Design review of the part shown in the three views and the two pictorial views. Dimensions are in mm from the part's minimum x, y and z. Coordinates: 2 decimals unless noted, no trailing zeros. Loops run counter-clockwise (first coordinate to the right, second up) from the corner with the lowest first, then second, coordinate; pieces in that order, holes last. Notation, with made-up numbers: M 55,-17.5 L 66,-17.5 A16 ccw 66,8.5 Z; hole C -20.5,-0.75 d4. An arc over 180 degrees is marked long. Use one line per item in the form item = value.
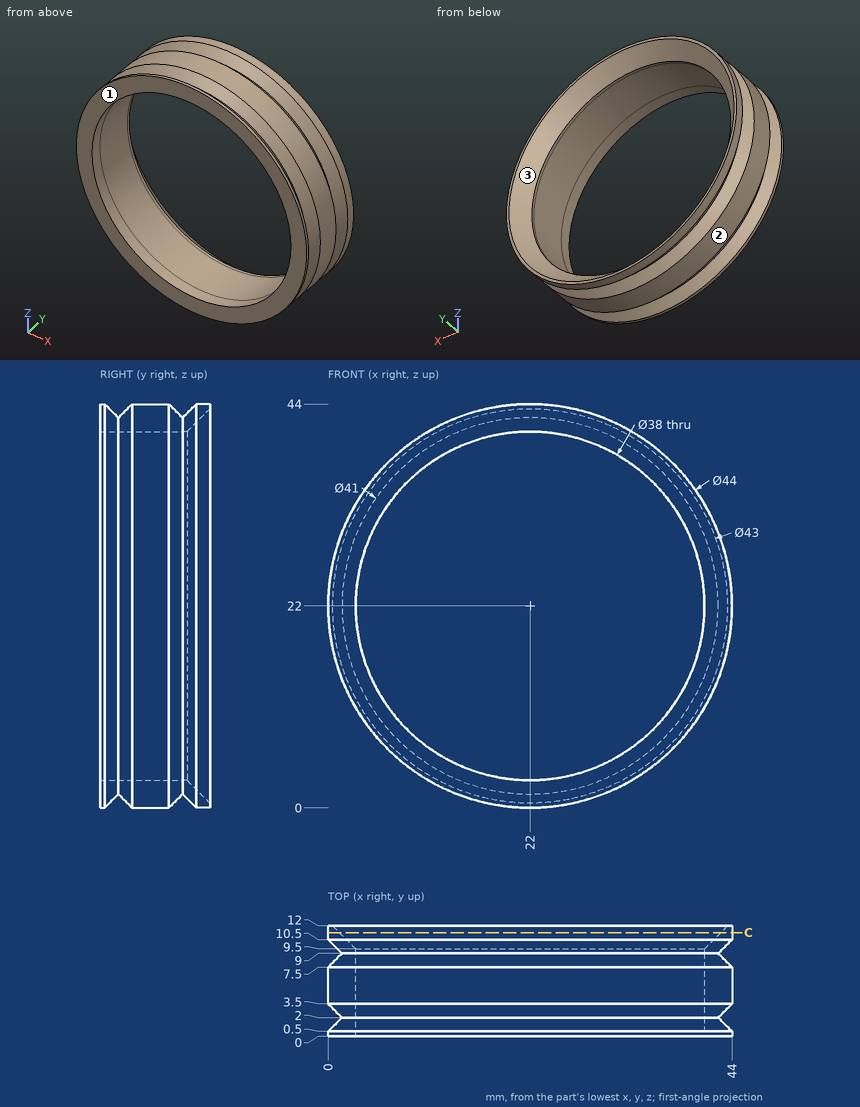
1. Add section C-C (y = 11.25). State the section outline as (x, z) points, then the cut area to 3 significant figures.
Response values:
outline = C 22,22 d44; hole C 22,22 d41.5
area = 168 mm^2
2. Wall thickness on line 1 along Z through (x, y) = (22, 6.5); line 2 along X through (y, z) = (2.25, 16); line 3 along X through (y, z) = (7.25, 21): over which ranges is each line inside the solid? List them lowest first. Write a range as from..to.
Response values:
line_1 = 0..3, 41..44
line_2 = 2.14..3.97, 40.03..41.86
line_3 = 0.02..3.03, 40.97..43.98
3. The part is to be moulded in two halves that separate along Z. For the marked faces 1, 2 and 3, say which applies: pulls with the +Z half, pulls with the -Z half, needs draft (parallel to the pull), parting line crosses it, or undercut.
Response values:
face_1 = needs draft
face_2 = parting line crosses it
face_3 = undercut
4. Insertion check: P1, Ø12, axis at x = 14.5, z = 25, coming from the -Y side; P2, Ø8, axis at x = 7, z = 13.5, coming from the +Y side. Each pin has a flat end and moves straight along its axis. Give the tip position at first contact, or say it passes through.
Response values:
P1 = through
P2 = 11.74
